Here's how the part is built. I have some questions about the finished solid (model axes, mm). Face numbers are marked on the shaded views. A direction names the side the tool comes from. Coordinates: 2 decimals unless noted, no trailing zeros. Write each loop counter-clockwise with the first axis right and the second up, starting at its lowest first coordinate (ties: lowest second). Pieces come first, ordered by that corner, then holes. Notation, with made-up numbers: M -18.75,50.25 L -7.75,50.25 A12 cw -7.75,62.25 Z; hole C 37,49.5 d8. An arc over 180 degrees is marked long. Use one line per item in the form item = value. Start each with the question number.
1. I'm going to push flat-ended pins straight in: pin 1 Ø5.5 at (x, y) = (-2, 1.5) entering from +Z; pin 2 Ø1.5 at (x, z) = (2, 8.5) entering from +Y; pin 3 Ø2 at (y, z) = (8.5, 12.5) entering from -X. Where does each tip first touch, or does it pass through?
2. Thinking about a two-plate mould opening in X: for the marked faces 4, 5, 6 and 7, which applies, released by +X, released by -X, zero draft, split by the parting line, or undercut?
3. Please list where these lines run through material, in increasing order: line 1 along Y through (x, z) = (0, 1); line 2 along Z through (x, y) = (1.5, -5); line 3 along Z through (x, y) = (-5, -4). Write a range as [from, to].
4. I want a section at D-D, the plane y = 8.75. List the corners of the cut face in (x, z) for me, plus the area to 3 significant figures.
5. I want a section at B-B, the plane z = 14. List the corners of the cut face in (x, y) for me, plus the area to 3 significant figures.
6. I want a section at A-A, the plane x = 0. List the corners of the cut face in (y, z) for me.
7. On a 3-axis mill with a long thin cutter (end or side, diameter ignored), from which of +Z, -Z, +X, -X, +Y, -Y can I reach the whole of each face in a straight line? I mean the marked faces 1, 2 and 3. Say none if no direction works.
from build123d import *

# Parameters (mm, degrees)
F0_R     = 12.25
F1_DEPTH = 20
F2_W     = 11
F2_H     = 11
F3_DEPTH = 10
F4_R     = 1.9
F5_DEPTH = 40
F6_R     = 6.75
F6_R_2   = 1.9
F7_DEPTH = 7
F8_SIZE  = 0.6


with BuildPart() as f1:
    # F0 (on Top) → F1 (new body)
    with BuildSketch(Plane.XY):
        Circle(F0_R)
    extrude(amount=F1_DEPTH)

    # F2 (on face) → F3 (cut)
    with BuildSketch(Plane.XY.offset(20)):
        Rectangle(F2_W, F2_H)
    extrude(amount=-F3_DEPTH, mode=Mode.SUBTRACT)

    # F4 (on face) → F5 (cut)
    with BuildSketch(Plane.XY.offset(10)):
        Circle(F4_R)
    extrude(amount=-F5_DEPTH, mode=Mode.SUBTRACT)

    # F6 (on face) → F7 (join)
    with BuildSketch(Plane(origin=(0, 0, 0), x_dir=(1, 0, 0), z_dir=(0, 0, -1))):
        Circle(F6_R)
        Circle(F6_R_2, mode=Mode.SUBTRACT)
    extrude(amount=F7_DEPTH)

    # F8
    f8_edges = [f1.edges().sort_by_distance(p)[0] for p in [
        (-6.75, 0, -7),
    ]]
    chamfer(f8_edges, length=F8_SIZE)


solid = f1.part
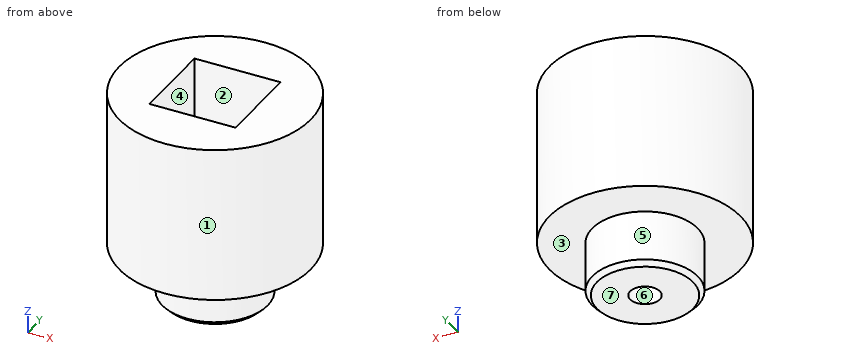
Answer list:
q1.pin_1 = 10
q1.pin_2 = 12.19
q1.pin_3 = -9.69
q2.face_4 = undercut
q2.face_5 = split by the parting line
q2.face_6 = undercut
q2.face_7 = zero draft
q3.line_1 = [-12.25, -1.9], [1.9, 12.25]
q3.line_2 = [-7, 10]
q3.line_3 = [-6.75, 10]
q4.outline = M -8.57,0 L 8.57,0 L 8.57,20 L -8.57,20 Z
q4.area = 343 mm²
q5.outline = C 0,0 d24.5; hole M -5.5,-5.5 L 5.5,-5.5 L 5.5,5.5 L -5.5,5.5 Z
q5.area = 350 mm²
q6.outline = M -12.25,0 L -6.75,0 L -6.75,-6.4 L -6.15,-7 L -1.9,-7 L -1.9,10 L -5.5,10 L -5.5,20 L -12.25,20 Z; M 1.9,-7 L 6.15,-7 L 6.75,-6.4 L 6.75,0 L 12.25,0 L 12.25,20 L 5.5,20 L 5.5,10 L 1.9,10 Z
q7.face_1 = +Z, -Z
q7.face_2 = +Z
q7.face_3 = -Z
